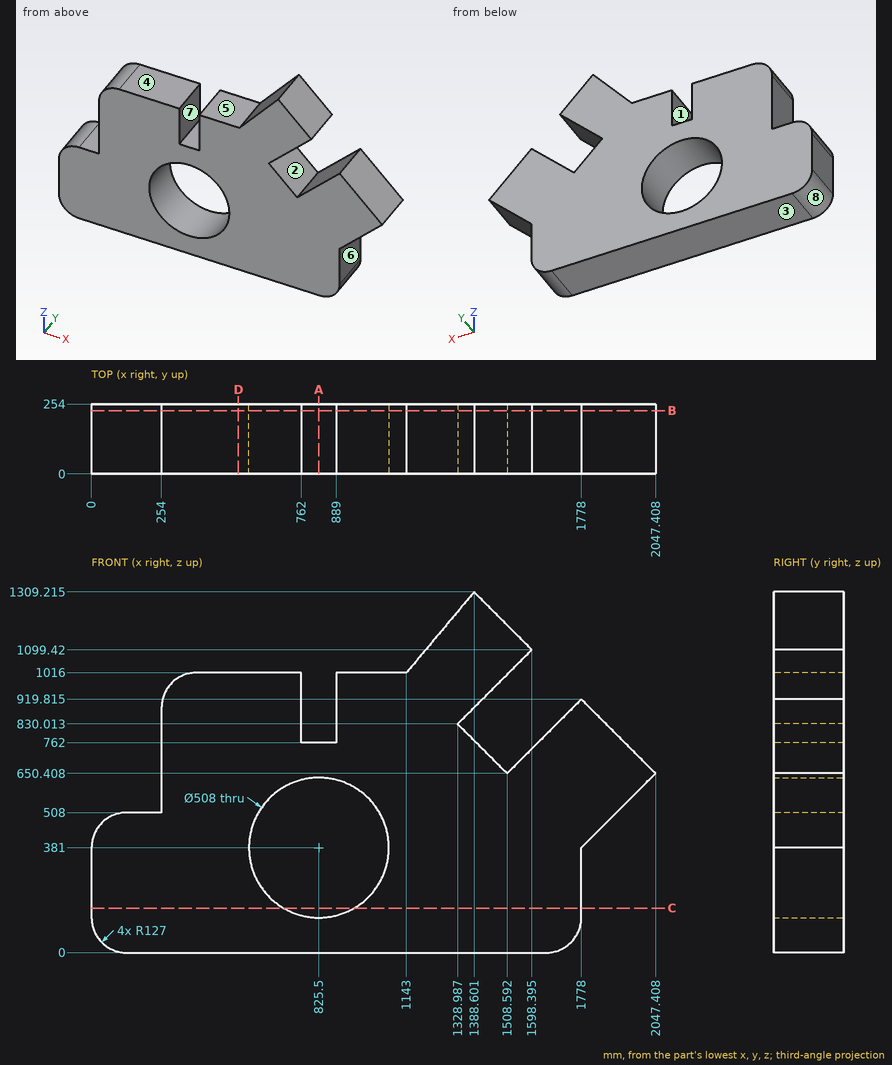
Print and shaded views of the part. All mm, measured from the part's lowest x, y and z. A direction names the side the tool comes from. Coordinates: 2 decimals unless noted, no trailing zeros. Loops run counter-clockwise (first coordinate to the right, second up) from the corner with the lowest first, then second, coordinate; pieces in that order, holes last. Notation, with made-up numbers: M 45.5,89.5 L 98.5,89.5 A20 cw 98.5,102.5 Z; hole C -20.5,69 d1. An arc over 180 degrees is marked long. Use a Markdown table: item, result. Add a question column.
Q1. Cut at B-B (y = 230). Write the cut outline in (x, z) (1 decimal).
Q2. Pin check, flat tips, straight feed: P1, Ø8, axis at y = 139, z = 777.5, coming from the +X side (1 decimal); P2, Ø1, axis at y = 195, z = 1095.5, coming from the -X side; P3, Ø3, axis at x = 839, y = 121, coming from the +Z side. Stop position of each tip, or through.
Q3. Cut at C-C (z = 161.5). Write the cut outline in (x, y), and give its area (3 significant figures).
Q4. Cut at D-D (x = 533.5). Write the cut outline in (y, z), and give its area (3 significant figures).
Q5. Which spindle directions (+Z, -Z, +X, -X, +Y, -Y) get a long thin tool onto all of the face, cutting with end or side? Do the marked faces 5, 6, 7 and 8. Say none if no direction does.
Q6. Cut at A-A (x = 825.5). Write the cut outline in (y, z), and give its area (3 significant figures).
Q7. Mould opens along Z. For the marked faces 1, 2, 3 and 4 say: +Z half, -Z half, draft (parallel to the pull), parting line (faces both ways), or undercut.
Q8. Probe L1, parallel to Z at x = 825.5, y = 166; L2, parallel to X at y = 244.5, z = 803 (1 decimal); L3, parallel to X at y = 95, z = 885.5 (1 decimal). List the from-to ranges inside material, lowest first.
Worked out:
| question | item | result |
|---|---|---|
| 1 | outline | M 0,127 A127 ccw 127,0 L 1651,0 A127 ccw 1778,127 L 1778,381 L 2047.4,650.4 L 1778,919.8 L 1508.6,650.4 L 1329,830 L 1598.4,1099.4 L 1388.6,1309.2 L 1143,1016 L 889,1016 L 889,762 L 762,762 L 762,1016 L 381,1016 A127 ccw 254,889 L 254,508 L 127,508 A127 ccw 0,381 Z; hole C 825.5,381 d508 |
| 2 | P1 | stops at x = 1924.3 |
| 2 | P2 | stops at x = 1209.17 |
| 2 | P3 | stops at z = 762 |
| 3 | outline | M 0,0 L 697.69,0 L 697.69,254 L 0,254 Z; M 953.31,0 L 1778,0 L 1778,254 L 953.31,254 Z |
| 3 | area | 387,000 mm2 |
| 4 | outline | M 0,0 L 254,0 L 254,1016 L 0,1016 Z |
| 4 | area | 258,000 mm2 |
| 5 | face 5 | +Z, -X, +Y, -Y |
| 5 | face 6 | -Z, +X, +Y, -Y |
| 5 | face 7 | +Z, +Y, -Y |
| 5 | face 8 | -Z, -X, +Y, -Y |
| 6 | outline | M 0,0 L 254,0 L 254,127 L 0,127 Z; M 0,635 L 254,635 L 254,762 L 0,762 Z |
| 6 | area | 64,500 mm2 |
| 7 | face 1 | draft |
| 7 | face 2 | undercut |
| 7 | face 3 | -Z half |
| 7 | face 4 | +Z half |
| 8 | L1 | z = 0 to 127, 635 to 762 |
| 8 | L2 | x = 254 to 762, 889 to 1356, 1661.2 to 1894.8 |
| 8 | L3 | x = 254 to 762, 889 to 1384.5, 1743.7 to 1812.3 |
